Source: CAD feature listing. Evaluate the final solid. Frame: model axes, mm. Round coordinates to 2 decimals unless told otherwise and drop trailing zeros. Write each loop counter-clockwise with the first axis right and the second up, starting at its lowest first coordinate (ties: lowest second). Pieces come first, ordered by that corner, then holes.
```python
from build123d import *

# Parameters (mm, degrees)
F1_DEPTH = 3


with BuildPart() as f1:
    # F0 (on Top) → F1 (new body)
    with BuildSketch(Plane.XY):
        with BuildLine():
            Line((44.865233, 76.85111), (-76.134767, 76.85111))
            ThreePointArc((-76.134767, 76.85111), (-77.54898, 76.265324), (-78.134767, 74.85111))
            Line((-78.134767, 74.85111), (-78.134767, -13.489018))
            ThreePointArc((-78.134767, -13.489018), (-77.389263, -15.046657), (-75.708528, -15.443071))
            Line((-75.708528, -15.443071), (-40.880867, -7.8461))
            ThreePointArc((-40.880867, -7.8461), (-39.749467, -7.146545), (-39.307105, -5.892048))
            Line((-39.307105, -5.892048), (-39.307105, 36.074161))
            Line((-39.307105, 36.074161), (-39.307105, 42.227437))
            Line((-39.307105, 42.227437), (-30.88689, 40.253897))
            Line((-30.88689, 40.253897), (-27.519081, 46.517927))
            Line((-27.519081, 46.517927), (-18.964279, 44.593372))
            Line((-18.964279, 44.593372), (-17.757622, 50.070808))
            Line((-17.757622, 50.070808), (-9.134416, 48.17115))
            Line((-9.134416, 48.17115), (-5.162104, 54.655201))
            Line((-5.162104, 54.655201), (3.258111, 52.681661))
            Line((3.258111, 52.681661), (4.549114, 58.189796))
            Line((4.549114, 58.189796), (12.969329, 56.216255))
            Line((12.969329, 56.216255), (14.260333, 61.72439))
            Line((14.260333, 61.72439), (22.680548, 59.75085))
            Line((22.680548, 59.75085), (24.824019, 65.569257))
            Line((24.824019, 65.569257), (33.244234, 63.595717))
            Line((33.244234, 63.595717), (47.234441, 76.85111))
            Line((47.234441, 76.85111), (44.865233, 76.85111))
        make_face()
    extrude(amount=F1_DEPTH)


solid = f1.part
```
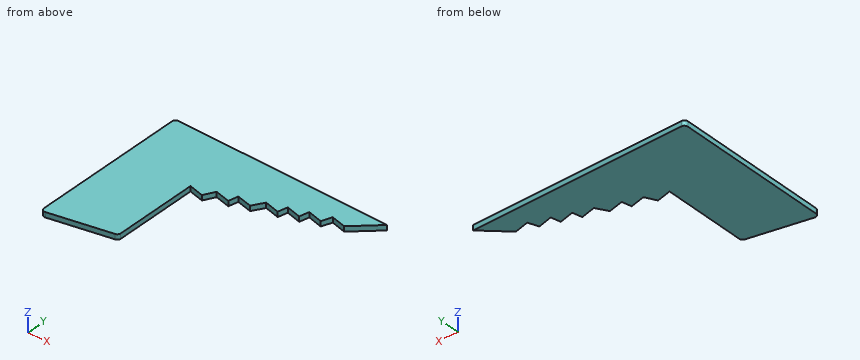
Q1. Section query A-A, the plane z = 1.55. Output: boundary loops of the cut face in (x, y), and give its area (3 significant figures).
Q2. Section query B-B, the plane y = 29. Output: boundary loops of the cut face in (x, z).
Q3. Line query: line 1 (X direction, y = 9.5, z = 1.45); line 2 (Y direction, x = -27, z = 0.5); line 3 (Y direction, x = -16, z = 2.65). Output: solid intervals per line, ascending.
Q4. Section query C-C, the plane x = -14.5. Output: boundary loops of the cut face in (y, z), and give its area (3 significant figures).
Filled in:
1. outline: (-78.13, -13.49) arc R2 ccw to (-75.71, -15.44) - (-40.88, -7.85) arc R2 ccw to (-39.31, -5.89) - (-39.31, 42.23) - (-30.89, 40.25) - (-27.52, 46.52) - (-18.96, 44.59) - (-17.76, 50.07) - (-9.13, 48.17) - (-5.16, 54.66) - (3.26, 52.68) - (4.55, 58.19) - (12.97, 56.22) - (14.26, 61.72) - (22.68, 59.75) - (24.82, 65.57) - (33.24, 63.6) - (47.23, 76.85) - (-76.13, 76.85) arc R2 ccw to (-78.13, 74.85) - close
1. area: 5,270 mm2
2. outline: (-78.13, 0) - (-39.31, 0) - (-39.31, 3) - (-78.13, 3) - close
3. line 1: x = -78.13 to -39.31
3. line 2: y = 46.4 to 76.85
3. line 3: y = 49.68 to 76.85
4. outline: (49.35, 0) - (76.85, 0) - (76.85, 3) - (49.35, 3) - close
4. area: 82.5 mm2
